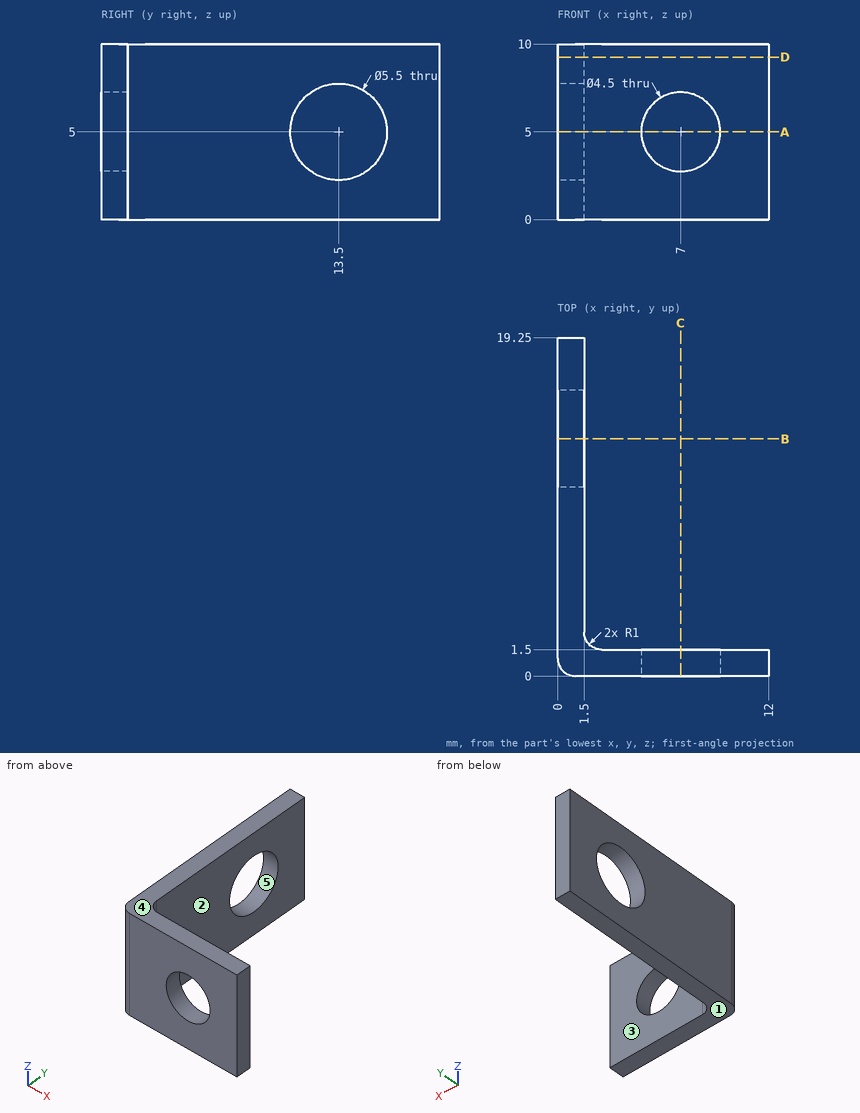
Geometry check sheet. Reference: drawing and pictorial views, mm from the part's lowest x, y, z. A direction names the side the tool comes from. Coordinates: 2 decimals unless noted, no trailing zeros. Order: outer loops, then holes, each group sorted by start corner. A loop starts at its lowest first (then second) coordinate and runs counter-clockwise, first axis right, second up. Notation, with made-up numbers: M 74,70 L 103,70 A35 ccw 103,109 Z; hole C 3.25,29 d4. An arc over 180 degrees is marked long. Write each question's results on one line, items separated by ' | '. Start each with the question number.
1. Material ranges on probe 1 along Z at (x, y) = (7, 0.75); probe 2 along X at (y, z) = (9.25, 5.5), recorded low to high.
2. Go/stop test with a flat-tipped pin: P1, Ø4, axis at y = 5.5, z = 2, coming from the +X side. Record where the tip stops, or that it passes through.
3. Cross-section at D-D on z = 9.25. Record the cut outline in (x, y), and give its area (3 significant figures).
4. Cross-section at B-B on y = 13.5. Record the cut outline in (x, z), and give its area (3 significant figures).
5. Cross-section at C-C on x = 7. Record the cut outline in (y, z), and give its area (3 significant figures).
6. Cross-section at A-A on z = 5. Record the cut outline in (x, y), and give its area (3 significant figures).
7. Mould release check, pull along Z, two halves, no side actions. Record for the marked faces 3, 4 and 5: +Z half, -Z half, draft (parallel to the pull), parting line (faces both ways), or undercut.
8. Access from +Z, -Z, +X, -X, +Y, -Y to the whole of each face (thin tool, end or side, straight path). Record for the marked faces 1 and 2.
Checks:
1) probe 1: z = 0 to 2.75, 7.25 to 10 | probe 2: x = 0 to 1.5
2) P1: stops at x = 1.5
3) outline: M 0,1 A1 ccw 1,0 L 12,0 L 12,1.5 L 2.5,1.5 A1 cw 1.5,2.5 L 1.5,19.25 L 0,19.25 Z | area: 44.6 mm²
4) outline: M 0,0 L 1.5,0 L 1.5,2.25 L 0,2.25 Z; M 0,7.75 L 1.5,7.75 L 1.5,10 L 0,10 Z | area: 6.75 mm²
5) outline: M 0,0 L 1.5,0 L 1.5,2.75 L 0,2.75 Z; M 0,7.25 L 1.5,7.25 L 1.5,10 L 0,10 Z | area: 8.25 mm²
6) outline: M 0,1 A1 ccw 1,0 L 4.75,0 L 4.75,1.5 L 2.5,1.5 A1 cw 1.5,2.5 L 1.5,10.75 L 0,10.75 Z; M 0,16.25 L 1.5,16.25 L 1.5,19.25 L 0,19.25 Z; M 9.25,0 L 12,0 L 12,1.5 L 9.25,1.5 Z | area: 29.6 mm²
7) face 3: draft | face 4: +Z half | face 5: undercut
8) face 1: -Z, +X, -X, +Y, -Y | face 2: +Z, -Z, +X, +Y
